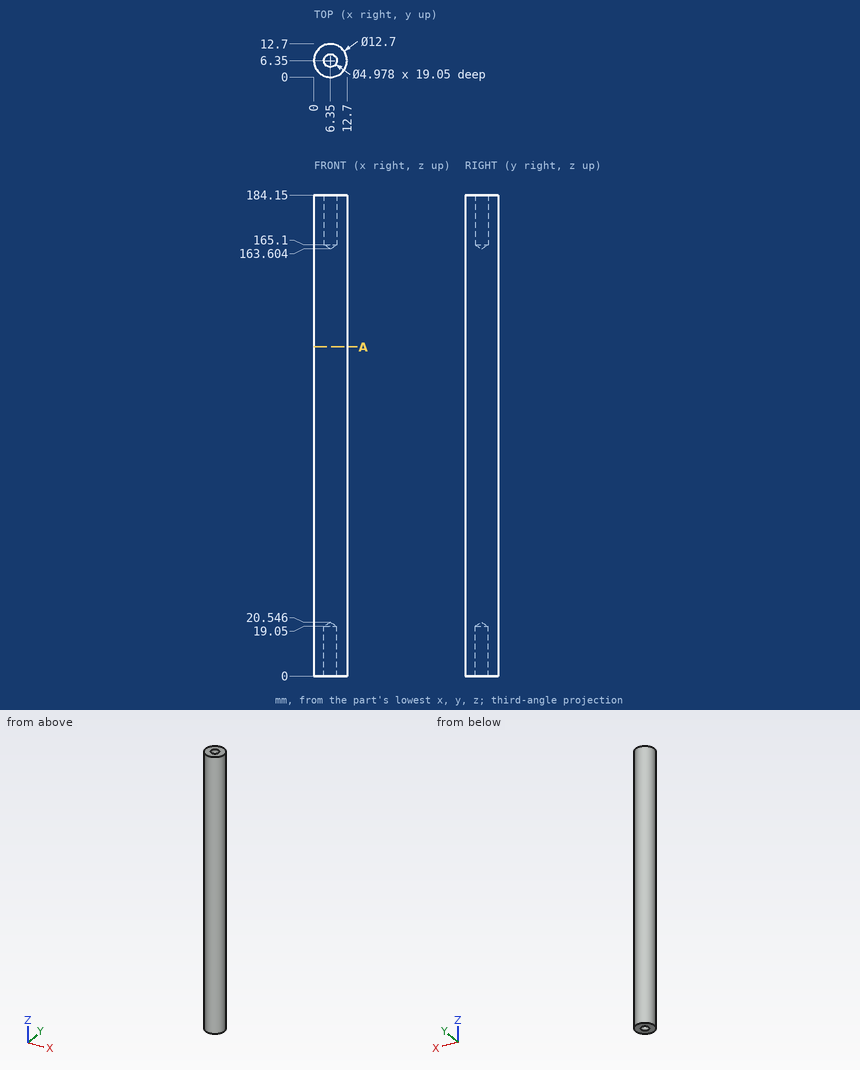
Answer from the drawing. Dimensions are ordinates in mm from the lowest x, y and z of the part. Coordinates: 2 decimals unless noted, no trailing zeros. Write each loop counter-clockwise with the first axis right and the second up, starting at its lowest first coordinate (ties: lowest second). Pieces come first, ordered by that corner, then holes. Notation, with made-up numbers: M 26.5,71.25 L 48.5,71.25 A29 cw 48.5,101.25 Z; hole C 9.5,47.5 d1. An arc over 180 degrees is marked long. Use one line per item in the form item = value. Start each with the question number.
1. The part is cut by section A-A (z = 126). Give the vertices of the cut face in (x, y), plus the area to 3 significant figures.
2. Straight lines are drawn through the part: probe 1 along Y at (x, z) = (6.35, 7.75); probe 2 along Y at (x, z) = (6.5, 136); probe 3 along X at (y, z) = (5, 77) (1 decimal). For each, find the intervals that lie inside material, in ascending order. Write a range as from..to.
3. Each of these flat-tipped pins is pushed along its axis until it touches: P1, Ø4.5, axis at x = 6.35, y = 6.35, coming from the +Z side; P2, Ø1.5, axis at y = 8.5, z = 53, coming from the -X side; P3, Ø1, axis at x = 5.5, y = 6.5, coming from the +Z side. Where does it stop, or does it pass through?
Evaluation:
q1.outline = C 6.35,6.35 d12.7
q1.area = 127 mm^2
q2.probe_1 = 0..3.86, 8.84..12.7
q2.probe_2 = 0..12.7
q2.probe_3 = 0.1..12.6
q3.P1 = 164.96
q3.P2 = 0.16
q3.P3 = 164.42
